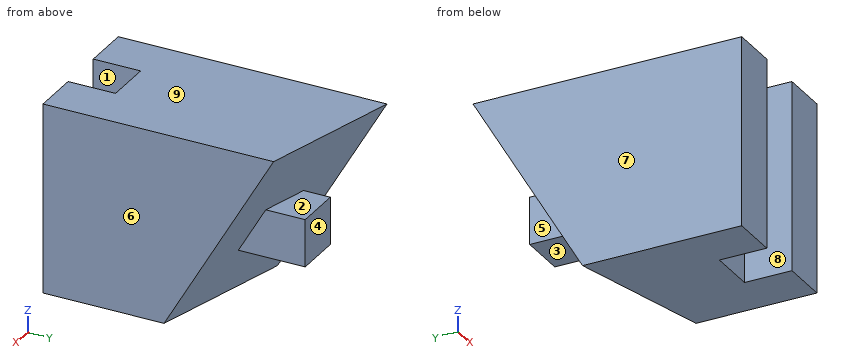
```python
from build123d import *

# Parameters (mm, degrees)
ESBO_O1_W                = 60
ESBO_O1_H                = 85
RESSALTO_EXTRUS_O1_DEPTH = 45
CORTE_EXTRUS_O1_REACH    = 102.9
ESBO_O7_W                = 70
ESBO_O7_H                = 90
RESSALTO_EXTRUS_O2_REACH = 108.066
ESBO_O8_W                = 15
ESBO_O8_H                = 15
CORTE_EXTRUS_O2_REACH    = 115.358
ESBO_O9_W                = 15
ESBO_O9_H                = 15


with BuildPart() as part:
    # Esboço1 → Ressalto-extrusão1 (new body)
    with BuildSketch(Plane(origin=(0, 0, 0), x_dir=(0, 0, -1), z_dir=(1, 0, 0))):
        with Locations((-30, 42.5)):
            Rectangle(ESBO_O1_W, ESBO_O1_H)
    extrude(amount=RESSALTO_EXTRUS_O1_DEPTH)

    # Esboço7 → Corte-extrusão1 (cut, up to next)
    with BuildSketch(Plane(origin=(9.603131429, 35.839374403, -20.691872459), x_dir=(-0.9741169476962972, 0.19576038710152016, -0.11302231218972801), z_dir=(-0.22604462437945605, -0.8436100229619508, 0.48705847384814865)), mode=Mode.PRIVATE) as corte_extrus_o1_sk1:
        with Locations((-10.222277995, -55.295886242)):
            Rectangle(ESBO_O7_W, ESBO_O7_H)
    corte_extrus_o1_tool1 = extrude(corte_extrus_o1_sk1.sketch, amount=-CORTE_EXTRUS_O1_REACH, mode=Mode.PRIVATE) & part.part
    add(corte_extrus_o1_tool1.solids().sort_by_distance((19.560826, 61.4862, 28.351115))[0], mode=Mode.SUBTRACT)

    # Ressalto-extrusão2: up to this plane
    ressalto_extrus_o2_end = Plane(origin=(9.603131429, 35.839374403, -20.691872459), z_dir=(-0.22604462437945594, -0.8436100229619508, 0.4870584738481487))
    # Esboço8 → Ressalto-extrusão2 (add, up to the surface)
    with BuildSketch(Plane(origin=(0, 75, 0), x_dir=(1, 0, 0), z_dir=(0, 1, 0)), mode=Mode.PRIVATE) as ressalto_extrus_o2_sk1:
        with Locations((22.5, -27.5)):
            Rectangle(ESBO_O8_W, ESBO_O8_H)
    ressalto_extrus_o2_tool1 = split(extrude(ressalto_extrus_o2_sk1.sketch, amount=-RESSALTO_EXTRUS_O2_REACH, mode=Mode.PRIVATE), bisect_by=ressalto_extrus_o2_end, keep=Keep.BOTH, mode=Mode.PRIVATE)
    add(ressalto_extrus_o2_tool1.solids().sort_by_distance((22.5, 75, 27.5))[0])

    # Esboço9 → Corte-extrusão2 (cut, up to next)
    with BuildSketch(Plane(origin=(0, 0, 0), x_dir=(-1, 0, 0), z_dir=(0, 0, -1)), mode=Mode.PRIVATE) as corte_extrus_o2_sk1:
        with Locations((-22.5, 7.5)):
            Rectangle(ESBO_O9_W, ESBO_O9_H)
    corte_extrus_o2_tool1 = extrude(corte_extrus_o2_sk1.sketch, amount=-CORTE_EXTRUS_O2_REACH, mode=Mode.PRIVATE) & part.part
    add(corte_extrus_o2_tool1.solids().sort_by_distance((22.5, 7.5, 0))[0], mode=Mode.SUBTRACT)


solid = part.part
```
Can you work these out from the model? Positions are in its coordinate system, mm. Face numbers are marked on the shaded views. A direction names the side the tool comes from. Coordinates: 2 decimals unless noted, no trailing zeros. Write each loop counter-clockwise with the first axis right and the second up, starting at its lowest first coordinate (ties: lowest second). Pieces come first, ordered by that corner, then holes. Notation, with made-up numbers: M 53.5,65.5 L 77.5,65.5 A17 cw 77.5,94.5 Z; hole C 56.25,69.5 d9. An arc over 180 degrees is marked long. Write item = value, one per line. Start each with the question number.
Q1. Thinking about a two-plate mould opening in X: for the marked faces 6, 7, 8 and 9, which applies, released by +X, released by -X, zero draft, split by the parting line, or undercut?
Q2. I'm going to push flat-ended pins straight in: pin 1 (12 mm diameter, centred on y = 66.5, z = 26.5, fed in from +X); pin 2 (16.5 mm diameter, centred on x = 19.5, z = 26.5, fed in from +Y); pin 3 (7.5 mm diameter, centred on x = 23.5, z = 43, fed in from -Y). Where does each tip first touch, or does it pass through?
Q3. If I drill on L1, parallel to X at y = 8, z = 30; L2, parallel to X at y = 62.5, z = 34; L3, parallel to Z at x = 7, y = 75, over which ranges is the centre line in solid material (lowest first)? Write a range as [from, to].
Q4. If we section it at C-C, the plane x = 16: Write out the boundary of the cut face in (y, z).
Q5. If we section it at B-B, the plane z = 27: Write out the boundary of the cut face in (x, y).
Q6. If we section it at A-A, the plane y = 12: Write out the boundary of the cut face in (x, z), then the cut area to 3 significant figures.
Q7. If we section it at D-D, the plane y = 74: Write out the boundary of the cut face in (x, z).
Q8. On a 3-axis mill with a long thin cutter (end or side, diameter ignored), from which of +Z, -Z, +X, -X, +Y, -Y can I reach the whole of each face in a straight line? I mean the marked faces 1, 2, 3, 4 and 5. Say none if no direction works.
Check sheet entries:
q1.face_6 = released by +X
q1.face_7 = released by -X
q1.face_8 = undercut
q1.face_9 = zero draft
q2.pin_1 = 30
q2.pin_2 = 75
q2.pin_3 = 15
q3.L1 = [0, 15], [30, 45]
q3.L2 = [0, 30]
q3.L3 = [45.93, 60]
q4.outline = M 15,0 L 46.07,0 L 57.62,20 L 75,20 L 75,35 L 66.28,35 L 80.71,60 L 15,60 Z
q5.outline = M 0,0 L 15,0 L 15,15 L 30,15 L 30,0 L 45,0 L 45,53.89 L 30,57.91 L 30,75 L 15,75 L 15,61.93 L 0,65.95 Z
q6.outline = M 0,0 L 15,0 L 15,60 L 0,60 Z; M 30,0 L 45,0 L 45,60 L 30,60 Z
q6.area = 1,800 mm²
q7.outline = M 0,40.95 L 41.05,60 L 0,60 Z; M 15,20 L 30,20 L 30,35 L 15,35 Z
q8.face_1 = +Z, -Z, -Y
q8.face_2 = +X, +Y
q8.face_3 = -Z, +X, +Y
q8.face_4 = -Z, +X, -X, +Y
q8.face_5 = -Z, +Y
